Here's the drawing with two shaded views (mm, measured from the low corner). I have some questions. A direction names the side the tool comes from. Give positions to 0.01 mm unless a question says otherwise; leave off trailing zeros. Loops run counter-clockwise (first coordinate to the right, second up) from the corner with the lowest first, then second, coordinate; pieces in that order, holes last. Notation, with made-up numbers: M 27,-26.75 L 72,-26.75 A12 ccw 72,-20.75 Z; hole C 42,30.5 d5. An arc over 180 degrees is marked long. Use a Markdown table: item, result. Add a question column.
1) If I drill on line 1 along Z through (x, y) = (1.75, 0.2); line 2 along Y through (x, z) = (4.5, 18.5); line 3 along X through (y, z) = (4, 15.5) (1 decimal), over which ranges is the centre line in solid material (lowest first)? Write a range as [from, to].
2) Suppose I cut it at D-D on x = 1. List the corners of the cut face in (y, z) for me, and give its area (3 significant figures).
3) Suppose I cut it at B-B on z = 12.5. List the corners of the cut face in (x, y) for me.
4) Suppose I cut it at A-A on x = 3.5. List the corners of the cut face in (y, z) for me (1 decimal).
5) Which directions (+Z, -Z, +X, -X, +Y, -Y) give clear straight access to the entire face, cutting with the end or side of a thin tool? Please do the marked faces 1, 2 and 3.
6) Will these pins go through, and if not, where does the flat tip stop? pin 1 Ø1.5 at (x, z) = (4, 5.5) entering from +Y; pin 2 Ø2 at (y, z) = (2, 16.5) entering from +X (1 decimal).
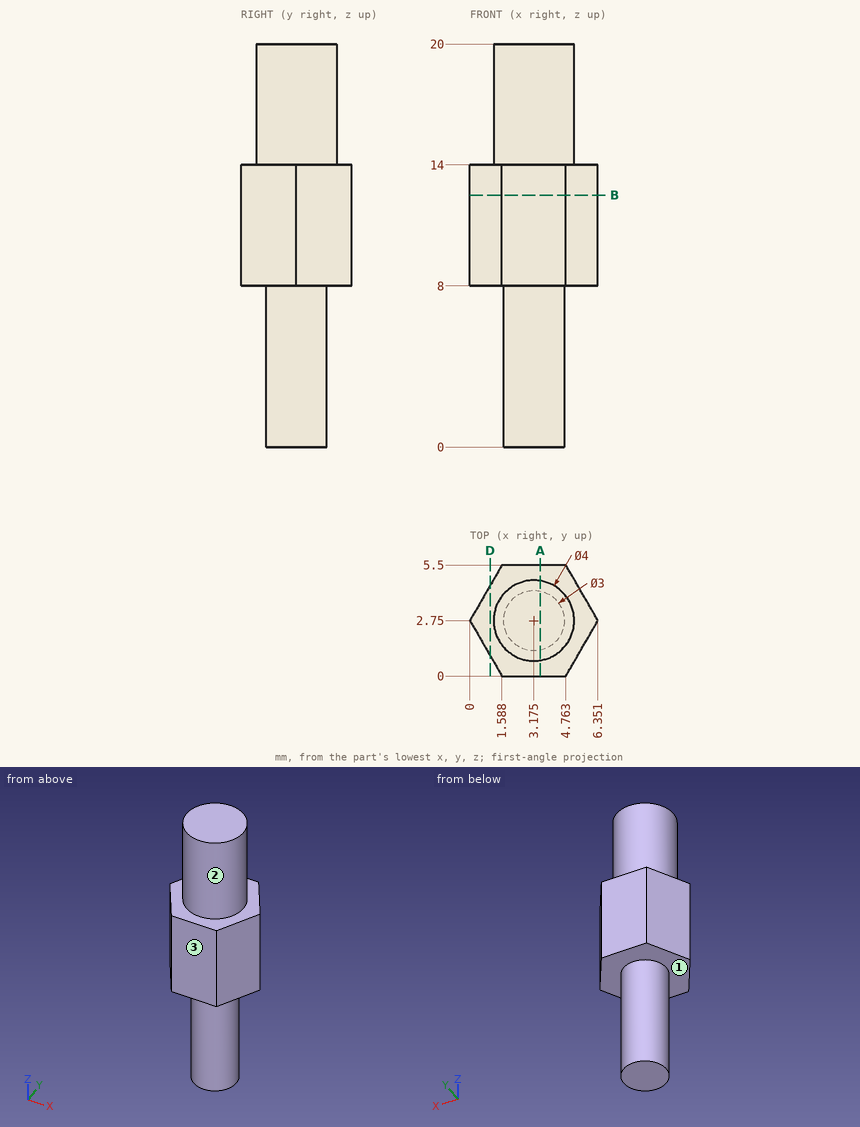
Answer block:
| question | item | result |
|---|---|---|
| 1 | line 1 | z = [8, 14] |
| 1 | line 2 | y = [1.25, 4.25] |
| 1 | line 3 | x = [1.6, 4.7] |
| 2 | outline | M 1.02,8 L 4.48,8 L 4.48,14 L 1.02,14 Z |
| 2 | area | 20.8 mm^2 |
| 3 | outline | M 0,2.75 L 1.59,0 L 4.76,0 L 6.35,2.75 L 4.76,5.5 L 1.59,5.5 Z |
| 4 | outline | M 0,8 L 1.3,8 L 1.3,0 L 4.2,0 L 4.2,8 L 5.5,8 L 5.5,14 L 4.7,14 L 4.7,20 L 0.8,20 L 0.8,14 L 0,14 Z |
| 5 | face 1 | -Z |
| 5 | face 2 | +Z |
| 5 | face 3 | +Z, -Z, +X, -X, -Y |
| 6 | pin 1 | stops at y = 4.25 |
| 6 | pin 2 | stops at x = 5.2 |
